```python
from build123d import *

# Parameters (mm, degrees)
F2_W     = 18
F2_H     = 1
F4_R     = 1.65
F5_DEPTH = 1
F6_R     = 1.65
F7_DEPTH = 35.001


with BuildPart() as f3:
    # F3: sweep along a path in F0
    with BuildLine(Plane.YZ) as f3_path:
        Line((-35, 0), (-5, 0))
        ThreePointArc((-5, 0), (-1.4644660941, 1.4644660941), (0, 5))
        Line((0, 5), (0, 115))
    # F2 (on plane+point) → F3 (sweep)
    with BuildSketch(Plane.XZ.offset(35)):
        with Locations((9, 0.5)):
            Rectangle(F2_W, F2_H)
    sweep(path=f3_path.line)

    # F4 (on face) → F5 (cut, through all)
    with BuildSketch(Plane.XY.offset(1)):
        with Locations((6, -14)):
            Circle(F4_R)
        with Locations((6, -28)):
            Circle(F4_R)
    extrude(amount=-F5_DEPTH, mode=Mode.SUBTRACT)

    # F6 (on face) → F7 (cut, through all)
    with BuildSketch(Plane(origin=(0, 0, 0), x_dir=(-1, 0, 0), z_dir=(0, 1, 0))):
        with Locations((-3, 24.4)):
            Circle(F6_R)
        with Locations((-14, 24.4)):
            Circle(F6_R)
        with Locations((-14, 101)):
            Circle(F6_R)
        with Locations((-3, 101)):
            Circle(F6_R)
        with BuildLine():
            Line((-18, 15), (-18, 0))
            Line((-18, 0), (-11, 0))
            Line((-11, 0), (-11, 13))
            ThreePointArc((-11, 13), (-11.5857864376, 14.4142135624), (-13, 15))
            Line((-13, 15), (-18, 15))
        make_face()
    extrude(amount=-F7_DEPTH, mode=Mode.SUBTRACT)


solid = f3.part
```
Verification items for the finished model (mm, model axes). A direction names the side the tool comes from. Coordinates: 2 decimals unless noted, no trailing zeros. Loops run counter-clockwise (first coordinate to the right, second up) from the corner with the lowest first, then second, coordinate; pieces in that order, holes last. Notation, with made-up numbers: (22, -25) -> (57, -25) arc R16 cw to (57, 1) -> close; hole circle Ø10 at (67.5, 35). An arc over 180 degrees is marked (long way). Answer in a Markdown table with one row per item. Add a question column.
1. Section check C-C, the plane z = 108.5. Enter the section's corners in (x, y).
2. Depth check by flat-ended pin: P1, Ø3.5, axis at x = 7.5, y = -20.5, coming from the +Z side; P2, Ø3, axis at x = 3, z = 101, coming from the -Y side; P3, Ø5.5, axis at x = 3, z = 24.4, coming from the -Y side. Enter the tip coordinate at first touch or a pass-through.
3. Access from +Z, -Z, +X, -X, +Y, -Y to the whole of each face (thin tool, end or side, straight path). Record for faces 1 (the face through (9, -1, 61)), 2 (the face through (6, -2, 1)), 3 (the face through (11, -12.2, 0.7)).
4. Section check B-B, the plane y = -28. Enter the section's corners in (x, z), then the cut area to 3 significant figures.
5. Section check D-D, the plane x = 6. Enter the section's corners in (y, z).
6. Draft check along Z on faces 4 (the face through (3.4, -0.5, 22.8)), 5 (the face through (5, -20, 0)), 6 (the face through (9, 0, 61)), 7 (the face through (5.423, -2.203, 2.141)). Enter one of: +Z half, -Z half, draft (parallel to the pull), parting line (faces both ways), or undercut.
7. Section check A-A, the plane x = 14. Enter the section's corners in (y, z), then the cut area to 3 significant figures.
8. Material ranges on probe 1 along X at (y, z) = (-0.7, 101); probe 2 along Y at (x, z) = (5, 42); probe 3 along Y at (x, z) = (6, 0.7), recorded low to high. Write a range as [from, to].
Derived:
| question | item | result |
|---|---|---|
| 1 | outline | (0, -1) -> (18, -1) -> (18, 0) -> (0, 0) -> close |
| 2 | P1 | stops at z = 1 |
| 2 | P2 | passes through |
| 2 | P3 | stops at y = -1 |
| 3 | face 1 | +Z, +X, -X, -Y |
| 3 | face 2 | -Z, +X, -X, +Y |
| 3 | face 3 | -Z, +X, +Y, -Y |
| 4 | outline | (0, 0) -> (4.35, 0) -> (4.35, 1) -> (0, 1) -> close; (7.65, 0) -> (11, 0) -> (11, 1) -> (7.65, 1) -> close |
| 4 | area | 7.70 mm² |
| 5 | outline | (-35, 0) -> (-29.65, 0) -> (-29.65, 1) -> (-35, 1) -> close; (-26.35, 0) -> (-15.65, 0) -> (-15.65, 1) -> (-26.35, 1) -> close; (-12.35, 0) -> (-5, 0) arc R5 ccw to (0, 5) -> (0, 115) -> (-1, 115) -> (-1, 5) arc R4 cw to (-5, 1) -> (-12.35, 1) -> close |
| 6 | face 4 | undercut |
| 6 | face 5 | -Z half |
| 6 | face 6 | draft |
| 6 | face 7 | +Z half |
| 7 | outline | (-1, 15) -> (0, 15) -> (0, 22.75) -> (-1, 22.75) -> close; (-1, 26.05) -> (0, 26.05) -> (0, 99.35) -> (-1, 99.35) -> close; (-1, 102.65) -> (0, 102.65) -> (0, 115) -> (-1, 115) -> close |
| 7 | area | 93.4 mm² |
| 8 | probe 1 | x = [0, 1.35], [4.65, 12.35], [15.65, 18] |
| 8 | probe 2 | y = [-1, 0] |
| 8 | probe 3 | y = [-35, -29.65], [-26.35, -15.65], [-12.35, -2.45] |
